Design review of the part built by this model. Coordinates are the model's own, in mm. Face numbers are marked on the shaded views. A direction names the side the tool comes from. Round coordinates to 2 decimals unless told otherwise and drop trailing zeros. Loops run counter-clockwise (first coordinate to the right, second up) from the corner with the lowest first, then second, coordinate; pieces in that order, holes last. Notation, with made-up numbers: M 88,56 L 101,56 A17 ccw 101,80 Z; hole C 49.5,42.5 d11. An arc over 180 degrees is marked long. Use a Markdown table: item, result.
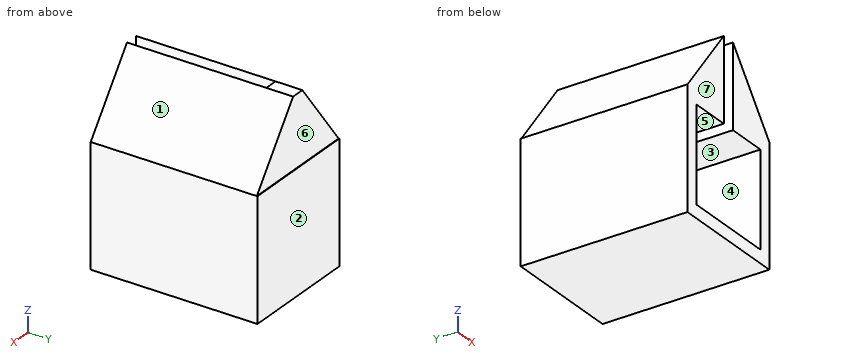
from build123d import *

# Parameters (mm, degrees)
F0_W      = 32.9184
F0_H      = 32.9184
F1_DEPTH  = 32.9184
F2_W      = 32.9184
F2_H      = 32.9184
F2_W_2    = 25.8064
F2_H_2    = 25.8064
F3_DEPTH  = 76.2
F4_W      = 3.7084
F4_H      = 76.2
F5_DEPTH  = 5.08
F7_DEPTH  = 76.2
F8_W      = 3.7084
F8_H      = 19.05
F9_DEPTH  = 7.3406
F10_DEPTH = 25.4
F11_DEPTH = 38.1


with BuildPart() as f1:
    # F0 (on Top) → F1 (new body)
    with BuildSketch(Plane.XY):
        with Locations((16.4592, -16.4592)):
            Rectangle(F0_W, F0_H)
    extrude(amount=F1_DEPTH)

    # F2 (on face) → F3 (join)
    with BuildSketch(Plane.XZ.offset(32.9184)):
        with Locations((16.4592, 16.4592)):
            Rectangle(F2_W, F2_H)
        with Locations((16.4592, 16.4592)):
            Rectangle(F2_W_2, F2_H_2, mode=Mode.SUBTRACT)
    extrude(amount=F3_DEPTH)

    # F4 (on face) → F5 (cut)
    with BuildSketch(Plane.XY.offset(32.9184)):
        with Locations((16.4592, -71.0184)):
            Rectangle(F4_W, F4_H)
    extrude(amount=-F5_DEPTH, mode=Mode.SUBTRACT)

    # F6 (on face) → F7 (join)
    with BuildSketch(Plane.XZ.offset(109.1184)):
        Polygon((0, 32.9184), (14.605, 32.9184), (14.605, 51.9684), align=None)
        Polygon((18.3134, 32.9184), (32.9184, 32.9184), (18.3134, 51.9684), align=None)
    extrude(amount=-F7_DEPTH)

    # F8 (on face) → F9 (join)
    with BuildSketch(Plane.XZ.offset(32.9184)):
        Polygon((18.3134, 51.9684), (18.3134, 32.9184), (32.9184, 32.9184), align=None)
        with Locations((16.4592, 42.4434)):
            Rectangle(F8_W, F8_H)
        Polygon((0, 32.9184), (14.605, 32.9184), (14.605, 51.9684), align=None)
    extrude(amount=-F9_DEPTH)

    # F10 (cut): a face of the model
    f10_faces = [f1.faces().sort_by_distance(p)[0] for p in [
        (16.4592, 0, 16.4592),
    ]]
    extrude(f10_faces, amount=-F10_DEPTH, mode=Mode.SUBTRACT)

    # F11 (cut): a face of the model
    f11_faces = [f1.faces().sort_by_distance(p)[0] for p in [
        (32.3032304578, -109.1184, 16.4592),
    ]]
    extrude(f11_faces, amount=-F11_DEPTH, mode=Mode.SUBTRACT)


solid = f1.part
1. Wall thickness on line 1 along X through (y, z) = (-58, 11); line 2 along Y through (x, z) = (28.5, 12.5); line 3 along Z through (x, y) = (10, -36.5): over which ranges is each line inside the solid? List them lowest first. Write a range as from..to.
Check values:
| item | result |
|---|---|
| line 1 | x = 0..3.56, 29.36..32.92 |
| line 2 | y = -32.92..-25.4 |
| line 3 | z = 0..3.56, 29.36..45.96 |
2. Machinability: for the marked faces 5, 6 and 7, which of the approach directions +Z, -Z, +X, -X, +Y, -Y give a long, thin tool a straight path to every point of the face, cutting with its end or side? Answer none if there is none.
Check values:
| item | result |
|---|---|
| face 5 | -Y |
| face 6 | +Z, +X, -X, +Y |
| face 7 | +Z, -Z, +X, -X, -Y |
3. The part is to be moulded in two halves that separate along Z. For the marked faces 1, 2, 3 and 4, say which applies: pulls with the +Z half, pulls with the -Z half, needs draft (parallel to the pull), parting line crosses it, or undercut.
Check values:
| item | result |
|---|---|
| face 1 | pulls with the +Z half |
| face 2 | needs draft |
| face 3 | undercut |
| face 4 | undercut |
4. Take a section at B-B on y = -66.5. Give the boundary of the cut face in (x, z) (3 decimals), and give its area (3 significant figures).
Check values:
| item | result |
|---|---|
| outline | M 0,0 L 32.918,0 L 32.918,32.918 L 18.313,51.968 L 18.313,29.362 L 29.362,29.362 L 29.362,3.556 L 3.556,3.556 L 3.556,29.362 L 14.605,29.362 L 14.605,51.968 L 0,32.918 Z |
| area | 683 mm² |
5. Take a section at D-D on y = -30. Give the boundary of the cut face in (x, z) (3 decimals), and give its area (3 significant figures).
Check values:
| item | result |
|---|---|
| outline | M 0,0 L 32.918,0 L 32.918,32.918 L 18.313,51.968 L 14.605,51.968 L 0,32.918 Z |
| area | 1,430 mm² |
6. Take a section at A-A on z = 11. Give the boundary of the cut face in (x, y).
Check values:
| item | result |
|---|---|
| outline | M 0,-71.02 L 3.56,-71.02 L 3.56,-32.92 L 29.36,-32.92 L 29.36,-71.02 L 32.92,-71.02 L 32.92,-25.4 L 0,-25.4 Z |
7. Insertion check: pin 1 (1.5 mm diameter, centred on y = -60, z = 40.5, fed in from -X); pin 2 (1 mm diameter, centred on x = 12, y = -65, fed in from +Z); pin 3 (15 mm diameter, centred on x = 11.5, z = 47, fed in from +Y). Each pin has a flat end and moves straight along its axis. Give the tip position at first contact, or say it passes through.
Check values:
| item | result |
|---|---|
| pin 1 | stops at x = 5.24 |
| pin 2 | stops at z = 49.22 |
| pin 3 | stops at y = -25.58 |
8. Take a section at C-C on x = 19.5. Give the boundary of the cut face in (y, z).
Check values:
| item | result |
|---|---|
| outline | M -71.02,0 L -25.4,0 L -25.4,32.92 L -25.58,32.92 L -25.58,50.42 L -71.02,50.42 L -71.02,29.36 L -32.92,29.36 L -32.92,3.56 L -71.02,3.56 Z |
